Autodesk Inventor part; units mm, degrees
ref_plane "작업 평면1" through (-20, 0, 0) normal (0, -1, 0) x (1, 0, 0)
ref_plane "YZ Plane" through (0, 0, 0) normal (1, 0, 0) x (0, 1, 0)
ref_plane "XZ Plane" through (0, 0, 0) normal (0, 1, 0) x (-1, 0, 0)
sketch "스케치1" plane through (0, 0, 0) normal (0, 0, 1) x (1, 0, 0)
  line L0 (-20, -25) -> (20, -25)
  line L1 (20, -25) -> (20, 25)
  line L2 (20, 25) -> (-20, 25)
  line L3 (-20, 25) -> (-20, -25)
  line L4 (-20, -25) -> (20, 25) construction
  line L5 (20, -25) -> (-20, 25) construction
  circle A0 centre (-15, 20) radius 1.5
  circle A1 centre (-15, -20) radius 1.5
  circle A2 centre (15, 20) radius 1.5
  circle A3 centre (15, -20) radius 1.5
  line L6 (0, 25) -> (0, -25)
  point P0 (0, 0)
  point P1 (-20, 0)
  dimension "d0" = 40
  dimension "d1" = 50
  dimension "d2" = 30
  dimension "d3" = 15
  dimension "d4" = 40
  dimension "d6" = 20
  dimension "d7" = 3
extrude "돌출1" add sketch "스케치1" along normal blind 5 contours L3 L2 L6 L0
sketch "스케치2" plane through (0, 0, 5) normal (0, 0, 1) x (1, 0, 0)
  circle A0 centre (15, -20) radius 1.5
  circle A1 centre (-15, -20) radius 1.5
  line L0 (0, 25) -> (-20, 25)
  line L1 (-20, 25) -> (-20, -25)
  line L2 (-20, -25) -> (0, -25)
  circle A2 centre (-15, 20) radius 1.5
  circle A3 centre (-15, -20) radius 1.5
  line L3 (-20, -25) -> (20, -25)
  line L4 (14, -15) -> (20, -15)
  line L5 (10, -25) -> (10, -19)
  arc A4 (14, -15) -> (10, -19) centre (14, -19) ccw
  line L6 (-28, 0) -> (28, 0)
  line L7 (0, -35) -> (0, 35)
  line L8 (-14, -15) -> (-20, -15)
  line L9 (-10, -25) -> (-10, -19)
  arc A5 (-10, -19) -> (-14, -15) centre (-14, -19) ccw
  line L10 (14, 15) -> (20, 15)
  line L11 (10, 25) -> (10, 19)
  arc A6 (10, 19) -> (14, 15) centre (14, 19) ccw
  line L12 (-10, 25) -> (-10, 19)
  arc A7 (-14, 15) -> (-10, 19) centre (-14, 19) ccw
  line L13 (-14, 15) -> (-20, 15)
  line L14 (0, -25) -> (0, 25)
  point P0 (10, -15)
  point P1 (0, 0)
  dimension "d13" = 10
  dimension "d16" = 4
extrude "돌출2" add sketch "스케치2" along normal blind 50 contours L7 L6 L1 L13 A7 L12 L0 | L7 L2 L9 A5 L8 L1 L6
fillet "모깎기1" radius 3 4 edges at (-15, -25, 5) (-20, -20, 5) (-15, 25, 5) (-20, 20, 5)
sketch "스케치3" plane through (-20, -25, 0) normal (-1, 0, 0) x (0, 0, 1)
  line L0 (2, 40) -> (55, 40)
  line L1 (5, 10) -> (55, 10)
  line L2 (4, 40) -> (12, 40)
  line L3 (12, 40) -> (12, 10)
  line L4 (12, 10) -> (4, 10)
  line L5 (4, 10) -> (4, 40)
  line L6 (0, 50) -> (0, 0)
  line L7 (12, 32) -> (4, 32)
  line L8 (4, 32) -> (4, 18)
  line L9 (4, 18) -> (12, 18)
  line L10 (12, 18) -> (12, 32)
  line L11 (12, 38) -> (4, 38)
  line L12 (4, 38) -> (4, 12)
  line L13 (4, 12) -> (12, 12)
  line L14 (12, 12) -> (12, 38)
  point P0 (0, 25)
  point P1 (15, 10)
  point P2 (12, 25)
  point P3 (4, 25)
  point P4 (12, 18)
  point P5 (12, 25)
  point P6 (8, 12)
  dimension "d17" = 8
  dimension "d18" = 4
  dimension "d21" = 8
  dimension "d28" = 26
extrude "돌출3" add sketch "스케치3" along normal blind 19 contours L11 L3 L7 L5 | L7 L3 L9 L5 | L9 L3 L13 L5
sketch "스케치5" plane through (-20, -13, 4) normal (0, -1, 0) x (1, 0, 0)
  circle A0 centre (-14, 4) radius 2.5
  line L0 (-19, 0) -> (-19, 8)
  point P0 (20, -4)
  point P1 (-19, 4)
  dimension "d29" = 5
  dimension "d30" = 5
extrude "돌출5" cut sketch "스케치5" against normal through all
ref_plane "작업 평면1" through (-20, 0, 0) normal (0, -1, 0) x (1, 0, 0)
sketch "스케치6" plane through (-20, 0, 0) normal (0, -1, 0) x (1, 0, 0)
  line L0 (0, 2) -> (0, 55)
  line L1 (0, 55) -> (-19, 55)
  line L2 (-19, 55) -> (-19, 47)
  line L3 (-19, 47) -> (0, 47)
  line L4 (0, 47) -> (0, 55)
  line L5 (-19, 12) -> (-19, 4)
  circle A0 centre (-14, 51) radius 2.5
  circle A1 centre (-14, 8) radius 2.5
  point P0 (20, 0)
  point P1 (0, 47)
  dimension "d31" = 0
  dimension "d33" = 8
  dimension "d34" = 8
  dimension "d35" = 4
extrude "돌출6" add sketch "스케치6" along normal mid plane 15 contours L3 L2 L1 L0
extrude "돌출7" cut sketch "스케치6" along normal mid plane 5 contours L3 L2 L1 L0
fillet "모깎기2" radius 4 4 edges at (-39, 5, 55) (-39, 5, 47) (-39, -5, 55) (-39, -5, 47)
equation "\"d3\" = 0.5 * d2"
equation "\"d34\" = d33"
equation "\"d35\" = 0.5 * d34"
properties part number "SuspensionSupporter"
CAD build for the part. Positions are in the model's coordinates, mm. A direction names the side the tool comes from. Give positions to 0.01 mm unless a question says otherwise; leave off trailing zeros. Write each loop counter-clockwise with the first axis right and the second up, starting at its lowest first coordinate (ties: lowest second). Pieces come first, ordered by that corner, then holes. Notation, with made-up numbers: (73, 50) -> (126, 50) arc R5 ccw to (126, 54) -> close; hole circle Ø11 at (-12, -18). An arc over 180 degrees is marked (long way). Return JSON: item names as keys, results as strings.
Item 1: Band-saw the part on B-B (x = -15). List the corners of the cut face in (y, z).
Answer below:
{"outline": "(-25, 0) -> (-21.5, 0) -> (-21.5, 5) -> (-22, 5) arc R3 ccw to (-25, 2) -> close; (-18.5, 0) -> (18.5, 0) -> (18.5, 5) -> (15, 5) -> (15, 55) -> (-15, 55) -> (-15, 5) -> (-18.5, 5) -> close; (21.5, 0) -> (25, 0) -> (25, 2) arc R3 ccw to (22, 5) -> (21.5, 5) -> close"}
Item 2: Band-saw the part on D-D (x = -34). List the corners of the cut face in (y, z), then the cut area to 3 significant figures.
Answer below:
{"outline": "(-13, 4) -> (13, 4) -> (13, 5.5) -> (-13, 5.5) -> close; (-13, 10.5) -> (13, 10.5) -> (13, 12) -> (-13, 12) -> close; (-7.5, 47) -> (-2.5, 47) -> (-2.5, 48.5) -> (-7.5, 48.5) -> close; (-7.5, 53.5) -> (-2.5, 53.5) -> (-2.5, 55) -> (-7.5, 55) -> close; (2.5, 47) -> (7.5, 47) -> (7.5, 48.5) -> (2.5, 48.5) -> close; (2.5, 53.5) -> (7.5, 53.5) -> (7.5, 55) -> (2.5, 55) -> close", "area": "108 mm2"}
Item 3: Tool access for faces 4 (the cylindrical face through (-14.93, -24.1, 4.14)), 5 (the flat face through (-28, 5, 47)), 6 (the flat face through (-29, -13, 8)), 7 (the flat face through (-29, 13, 8)), 8 (the flat face through (-13.5, 18.5, 5)): list every direction of +Z, -Z, +X, -X, +Y, -Y with a clear straight run to the whole face (end or side of a thin tool).
Answer below:
{"face 4": "+Z, -X, -Y", "face 5": "-X, +Y, -Y", "face 6": "+Z, -Z, -X, -Y", "face 7": "+Z, -Z, -X, +Y", "face 8": "+Z, -X, +Y"}
Item 4: Band-saw the part on A-A (y = 20). List the corners of the cut face in (x, z), then the cut area to 3 significant figures.
Answer below:
{"outline": "(-20, 0) -> (-16.5, 0) -> (-16.5, 5) -> (-17, 5) arc R3 ccw to (-20, 2) -> close; (-13.5, 0) -> (0, 0) -> (0, 55) -> (-10, 55) -> (-10, 5) -> (-13.5, 5) -> close", "area": "583 mm2"}
Item 5: Drop flat-ended pins along their axis: pin 1 (6.5 mm diameter, centred on y = 22.5, z = 23, fed in from -X); pin 2 (3 mm diameter, centred on y = 0, z = 34.5, fed in from -X); pin 3 (1.5 mm diameter, centred on x = -18.5, z = 20.5, fed in from -Y); pin 4 (2.5 mm diameter, centred on x = -15, y = -20, fed in from -Z). Give the stop position or say it passes through.
Answer below:
{"pin 1": "stops at x = -10", "pin 2": "stops at x = -20", "pin 3": "stops at y = -15", "pin 4": "passes through"}
Item 6: Band-saw the part on C-C (y = -12). List the corners of the cut face in (x, z).
Answer below:
{"outline": "(-39, 4) -> (-20, 4) -> (-20, 0) -> (0, 0) -> (0, 55) -> (-20, 55) -> (-20, 12) -> (-39, 12) -> close; hole circle Ø5 at (-34, 8)"}
Item 7: Two-plate mould, pull along Y, no slides. Class faces 1 (the flat face through (-28, -2.5, 51)), 2 (the cylindrical face through (-34.54, -4.96, 53.44)), 3 (the flat face through (-17, 15, 28)): +Y half, -Y half, draft (parallel to the pull), parting line (faces both ways), or undercut.
Answer below:
{"face 1": "undercut", "face 2": "draft", "face 3": "+Y half"}
Item 8: Drill centre lines: probe 1 along Z at (x, y) = (-34, 7.25); probe 2 along X at (y, z) = (-9, 37); probe 3 along X at (y, z) = (22.5, 15). Where is each one in solid material? Low to high.
Answer below:
{"probe 1": "z = 4 to 5.5, 10.5 to 12, 47 to 48.5, 53.5 to 55", "probe 2": "x = -20 to 0", "probe 3": "x = -10 to 0"}
